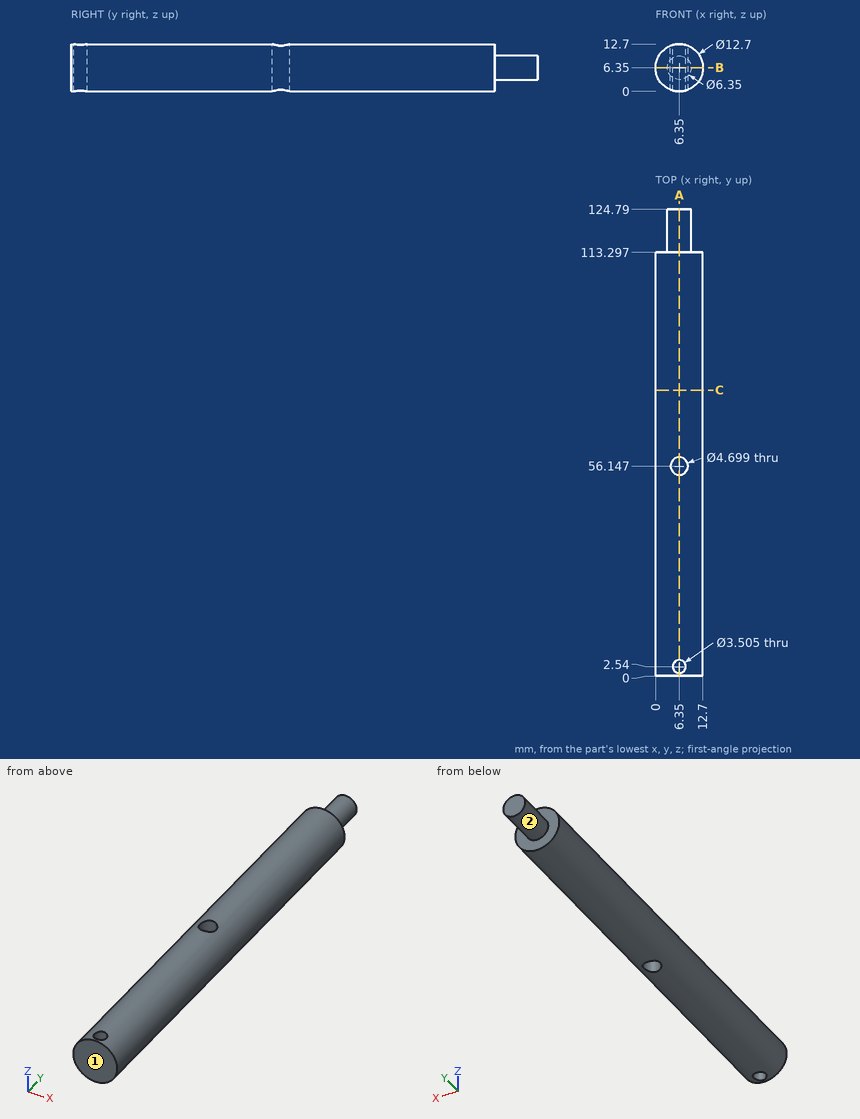
Source: three-view drawing plus pictorial views. Frame: mm from the lowest corner of the part. A direction names the side the tool comes from. Round coordinates to 2 decimals unless told otherwise and drop trailing zeros. Loops run counter-clockwise (first coordinate to the right, second up) from the corner with the lowest first, then second, coordinate; pieces in that order, holes last. Notation, with made-up numbers: (-39, -15.5) -> (-19, -15.5) arc R20 cw to (-19, 15.5) -> close; hole circle Ø3 at (66.25, 53). An arc over 180 degrees is marked (long way). Use one line per item in the form item = value.
Item 1: Contact query for flat-ended pins moving along their axis: pin 1 Ø4 at (y, z) = (28.5, 2) entering from -X; pin 2 Ø4 at (x, y) = (2, 79) entering from +Z; pin 3 Ø3 at (x, y) = (6.35, 2.54) entering from -Z; pin 4 Ø1 at (x, y) = (4.5, 79) entering from +Z (1 decimal). Output: stop coordinate, or through.
Evaluation:
pin_1 = 0.45
pin_2 = 12.25
pin_3 = through
pin_4 = 12.6
Item 2: Access query for the marked faces 1 and 2. Directions: +Z, -Z, +X, -X, +Y, -Y. A direction counts if a zero-diameter tool reaches every point of the face in a straight line with its end or side. Return the directions, or none.
Evaluation:
face_1 = +Z, -Z, +X, -X, -Y
face_2 = +Y
Item 3: Cut plane B-B on z = 6.35. Give the number of separate pieces and of enclosed holes in the cut face, then the cut area to 4 significant figures.
Evaluation:
separate_pieces = 1
enclosed_holes = 2
area = 1,485 mm2
Item 4: Cut plane A-A on x = 6.35. Output: boundary loops of the cut face in (y, z) (1 decimal).
Evaluation:
outline = (0, 0) -> (0.8, 0) -> (0.8, 12.7) -> (0, 12.7) -> close; (4.3, 0) -> (53.8, 0) -> (53.8, 12.7) -> (4.3, 12.7) -> close; (58.5, 0) -> (113.3, 0) -> (113.3, 3.2) -> (124.8, 3.2) -> (124.8, 9.5) -> (113.3, 9.5) -> (113.3, 12.7) -> (58.5, 12.7) -> close
Item 5: Material intervals for probe 1 along X at (y, z) = (2.54, 6.5); probe 2 along Y at (x, z) = (7.25, 6) (1 decimal); probe 3 along Y at (x, z) = (5, 1.75) (1 decimal), sorted ascending.
Evaluation:
probe_1 = 0 to 4.6, 8.1 to 12.7
probe_2 = 0 to 1, 4 to 54, 58.3 to 124.8
probe_3 = 0 to 1.4, 3.7 to 54.2, 58.1 to 113.3
Item 6: Cut plane C-C on y = 76.5. Output: boundary loops of the cut face in (x, z), then the cut area to 3 significant figures.
Evaluation:
outline = circle Ø12.7 at (6.35, 6.35)
area = 127 mm2
